```python
from build123d import *

# Parameters (mm, degrees)
SKETCH033_R  = 5
PAD010_DEPTH = 15
SKETCH035_R  = 2.7
PAD011_DEPTH = 18


with BuildPart() as part:
    # Sketch032 → AdditiveLoft section 0
    with BuildSketch(Plane.XY):
        with BuildLine():
            ThreePointArc((10, 50), (0, 60), (-10, 50))
            Line((-10, 50), (-10, -50))
            ThreePointArc((-10, -50), (0, -60), (10, -50))
            Line((10, 50), (10, -50))
        make_face()
    # Sketch034 → AdditiveLoft section 1
    with BuildSketch(Plane(origin=(0, 0, 5), x_dir=(0.984808, 0, -0.173648), z_dir=(0.173648, 0, 0.984808))):
        with BuildLine():
            ThreePointArc((10, 50), (0, 60), (-10, 50))
            Line((-10, 50), (-10, -50))
            ThreePointArc((-10, -50), (0, -60), (10, -50))
            Line((10, 50), (10, -50))
        make_face()
    loft()

    # Sketch033 (on Face3 of AdditiveLoft) → Pad010 (new body)
    with BuildSketch(Plane(origin=(0.85505, 0, 4.849232), x_dir=(0.984808, 0, -0.173648), z_dir=(0.173648, 0, 0.984808))):
        with Locations((0, 50)):
            Circle(SKETCH033_R)
        with Locations((0, -50)):
            Circle(SKETCH033_R)
        Circle(SKETCH033_R)
    extrude(amount=PAD010_DEPTH)

    # Sketch035 (on Face3 of AdditiveLoft) → Pad011 (join)
    with BuildSketch(Plane(origin=(0.85505, 0, 4.849232), x_dir=(0.984808, 0, -0.173648), z_dir=(0.173648, 0, 0.984808))):
        with Locations((0, 50)):
            Circle(SKETCH035_R)
        with Locations((0, -50)):
            Circle(SKETCH035_R)
        Circle(SKETCH035_R)
    extrude(amount=PAD011_DEPTH)


solid = part.part
```
The listing builds one solid part. Answer for the finished solid, in the listing's coordinates (mm). Give positions to 0.01 mm unless a question says otherwise; leave off trailing zeros. Loops run counter-clockwise (first coordinate to the right, second up) from the corner with the lowest first, then second, coordinate; pieces in that order, holes last. Notation, with made-up numbers: (-31, -19) - (-17, -19) arc R25 ccw to (-17, -2) - close; hole circle Ø7 at (31, 46.25). An arc over 180 degrees is marked (long way). Return JSON: item names as keys, results as strings. Group by question number.
1. Determine the mould class of faces 1 (the flat face through (0, 1, 0)), 2 (the cylindrical face through (6.253, 0.811, 20.631)), 3 (the flat face through (9.923, -0.7, 1.655)) for opening direction Z: pulls with the +Z half, pulls with the -Z half, needs draft (parallel to the pull), parting line crosses it, or undercut.
2. Find section A-A (y = 14). Write down the section's boundary in (x, z).
3. Straight lines are drawn through the part: line 1 (Y direction, x = -2, z = 5.5); line 2 (Y direction, x = 5.5, z = 11.5); line 3 (Z direction, x = -4.5, y = -35.5). For each, find the intervals that lie inside material, in ascending order. Write a range as [from, to].
4. Find section B-B (z = 12). State how many separate pieces and enclosed holes the cut face has, then the cut area to 3 significant figures.
5. Given pin 1 Ø8 at (x, z) = (-3, 16) entering from -Y; pin 2 Ø1 at (y, z) = (-27, 2.5) entering from -X; pin 3 Ø4 at (x, y) = (7.5, -40) entering from -Z; pin 4 Ø5 at (x, z) = (2.5, 13.5) entering from +Y, each flat-ended and moving along its own axis, determine where each tip first touches the part or whether it passes through.
Verdict:
{
 "1": {"face 1": "pulls with the -Z half", "face 2": "undercut", "face 3": "pulls with the +Z half"},
 "2": {"outline": "(-10, 0) - (10, 0) - (9.85, 3.26) - (-9.85, 6.74) - close"},
 "3": {"line 1": "y = [-54.06, -45.94], [-4.06, 4.06], [45.94, 54.06]", "line 2": "y = [-53.65, -46.35], [-3.65, 3.65], [46.35, 53.65]", "line 3": "z = [0, 5.79]"},
 "4": {"separate pieces": "3", "enclosed holes": "0", "area": "239 mm^2"},
 "5": {"pin 1": "stops at y = -54.69", "pin 2": "stops at x = -9.95", "pin 3": "stops at z = 0", "pin 4": "stops at y = 55"}
}
